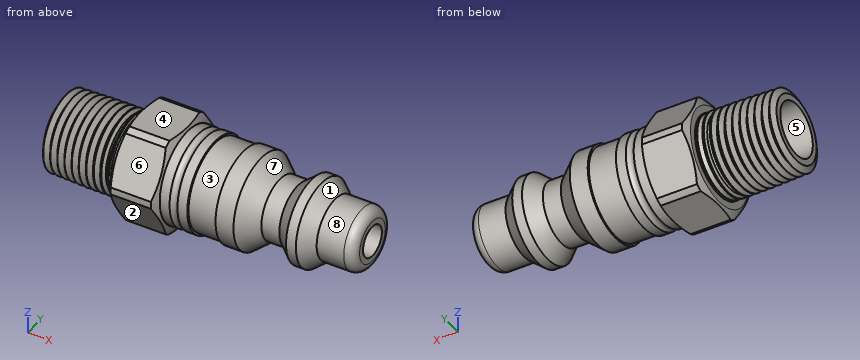
```python
from build123d import *

# Parameters (mm, degrees)
SKETCH6_W      = 11.300333551
SKETCH6_H      = 15.496408613
EXTRUDE1_DEPTH = 6.13324
FILLET1_R      = 1.27


with BuildPart() as part:
    # Sketch1 → Revolve1 (revolve)
    with BuildSketch(Plane.XY):
        Polygon((0, 0), (0, 4.202548436), (0.016953331, 4.234153018), (0.42773912, 4.999944315), (0.463586157, 5.001064591), (0.921387979, 4.262418014), (0.957235016, 4.26353829), (1.368020805, 5.029329586), (1.403867842, 5.030449862), (1.861669664, 4.291803285), (1.897516701, 4.292923561), (2.30830249, 5.058714857), (2.344149527, 5.059835133), (2.801951349, 4.321188556), (2.837798386, 4.322308832), (3.248584175, 5.088100128), (3.284431212, 5.089220404), (3.742233034, 4.350573827), (3.778080071, 4.351694103), (4.18886586, 5.1174854), (4.224712897, 5.118605675), (4.682514719, 4.379959098), (4.718361756, 4.381079374), (5.129147545, 5.146870671), (5.164994582, 5.147990947), (5.622796404, 4.409344369), (5.658643441, 4.410464645), (6.06942923, 5.176255942), (6.105276267, 5.177376218), (6.563078089, 4.43872964), (6.598925126, 4.439849916), (7.009710915, 5.205641213), (7.045557952, 5.206761489), (7.503359774, 4.468114911), (7.539206811, 4.469235187), (7.9499926, 5.235026484), (7.985839637, 5.23614676), (8.443641459, 4.497500182), (8.479488496, 4.498620458), (8.890274285, 5.264411755), (8.926121322, 5.265532031), (9.383923144, 4.526885454), (9.419770181, 4.528005729), (9.83055597, 5.293797026), (9.866403007, 5.294917302), (10.324204829, 4.556270725), (10.360051866, 4.557391001), (10.770837655, 5.323182297), (10.806684692, 5.324302573), (11.264486514, 4.585655996), (11.300333551, 4.586776272), (11.300333551, 0), align=None)
    revolve(axis=Axis((0, 0, 0), (-1, 0, 0)))

    # Sketch5 → Cut-Revolve2 (revolve, cut)
    with BuildSketch(Plane.XY, mode=Mode.PRIVATE) as cut_revolve2_sk:
        Polygon((9.96696, 0), (9.96696, 5.298059865), (11.300333551, 5.339729871), (11.300333551, 0), align=None)
    revolve(cut_revolve2_sk.sketch.rotate(Axis((0, 0, 0), (-1, 0, 0)), 180), axis=Axis((0, 0, 0), (-1, 0, 0)), mode=Mode.SUBTRACT)

    # Sketch6 → Cut-Revolve3 (revolve, cut)
    with BuildSketch(Plane.XY, mode=Mode.PRIVATE) as cut_revolve3_sk:
        with Locations((5.650166776, 12.891704307)):
            Rectangle(SKETCH6_W, SKETCH6_H)
    revolve(cut_revolve3_sk.sketch.rotate(Axis((0, 0, 0), (1, 0, 0)), 180), axis=Axis((0, 0, 0), (1, 0, 0)), mode=Mode.SUBTRACT)

    # Sketch7 → Revolve2 (revolve)
    with BuildSketch(Plane.XY, mode=Mode.PRIVATE) as revolve2_sk:
        Polygon((6.7056, 4.202548436), (9.96696, 5.1435), (9.96696, 4.202548436), align=None)
    revolve(revolve2_sk.sketch.rotate(Axis((0, 0, 0), (1, 0, 0)), 180), axis=Axis((0, 0, 0), (1, 0, 0)))

    # Sketch8 → Extrude1 (add)
    with BuildSketch(Plane(origin=(9.96696, 0, 0), x_dir=(0, 0, -1), z_dir=(1, 0, 0))):
        Polygon((0, 7.332348419), (-6.35, 3.666174209), (-6.35, -3.666174209), (0, -7.332348419), (6.35, -3.666174209), (6.35, 3.666174209), align=None)
    extrude(amount=EXTRUDE1_DEPTH)

    # Sketch9 → Cut-Revolve4 (revolve, cut)
    with BuildSketch(Plane.XY, mode=Mode.PRIVATE) as cut_revolve4_sk:
        Polygon((16.1002, 6.062348419), (15.626431419, 7.078348419), (10.440728581, 7.078348419), (9.96696, 6.062348419), (9.96696, 7.332348419), (16.1002, 7.332348419), align=None)
    revolve(cut_revolve4_sk.sketch.rotate(Axis((0, 0, 0), (1, 0, 0)), 180), axis=Axis((0, 0, 0), (1, 0, 0)), mode=Mode.SUBTRACT)

    # Sketch10 → Revolve3 (revolve)
    with BuildSketch(Plane.XY):
        with BuildLine():
            Line((16.1002, 0), (39.9, 0))
            Line((39.9, 0), (39.9, 3.96875))
            Line((39.9, 3.96875), (35.1375, 3.96875))
            Line((35.1375, 3.96875), (33.362408616, 5.458228526))
            Line((33.362408616, 5.458228526), (32.092408616, 5.458228526))
            Line((32.092408616, 5.458228526), (30.317317232, 3.96875))
            Line((30.317317232, 3.96875), (28.0001, 3.96875))
            Line((28.0001, 3.96875), (25.619597791, 5.966228526))
            Line((25.619597791, 5.966228526), (23.302380559, 5.966228526))
            Line((23.302380559, 5.966228526), (23.302380559, 5.712228526))
            Line((23.302380559, 5.712228526), (19.6562, 5.712228526))
            Line((19.6562, 5.712228526), (19.6562, 5.966228526))
            Line((19.6562, 5.966228526), (18.3862, 5.966228526))
            ThreePointArc((18.3862, 5.966228526), (17.8782, 5.712228526), (17.3702, 5.966228526))
            Line((17.3702, 5.966228526), (16.1002, 5.966228526))
            Line((16.1002, 5.966228526), (16.1002, 0))
        make_face()
    revolve(axis=Axis((0, 0, 0), (-1, 0, 0)))

    # Fillet1
    fillet1_edges = [part.edges().sort_by_distance(p)[0] for p in [
        (39.9, -3.96875, 0),
    ]]
    fillet(fillet1_edges, radius=FILLET1_R)

    # Sketch11 → Cut-Revolve5 (revolve, cut)
    with BuildSketch(Plane.XY, mode=Mode.PRIVATE) as cut_revolve5_sk:
        Polygon((9.96696, 3.4163), (16.1002, 1.984375), (39.9, 1.984375), (39.9, 0), (6.7056, 0), (0, 0), (0, 3.4163), align=None)
    revolve(cut_revolve5_sk.sketch.rotate(Axis((0, 0, 0), (-1, 0, 0)), 180), axis=Axis((0, 0, 0), (-1, 0, 0)), mode=Mode.SUBTRACT)


solid = part.part
```
Model file for the job. Use its own axes, mm. Face numbers are marked on the shaded views. A direction names the side the tool comes from. Coordinates: 2 decimals unless noted, no trailing zeros. Order: outer loops, then holes, each group sorted by start corner. A loop starts at its lowest first (then second) coordinate and runs counter-clockwise, first axis right, second up. Notation, with made-up numbers: (41.25, 6.5) -> (49.25, 6.5) arc R20 cw to (49.25, 35.5) -> close; hole circle Ø5 at (-10.75, 23). An arc over 180 degrees is marked (long way). Answer as a JSON object with one key per item and string values. Group by question number.
1) Pull direction X, two halves, no side cores. Call the marked faces 1, 2 and 3: +X half, -X half, draft (parallel to the pull), parting line (faces both ways), or undercut.
2) Which spindle directions (+Z, -Z, +X, -X, +Y, -Y) get a long thin tool onto all of the face, cutting with end or side? Do the marked faces 4, 5, 6, 7 and 8. Say none if no direction does.
3) Drill centre lines: L1, parallel to Y at x = 32.5, z = 3.75; L2, parallel to X at y = -3.25, z = 2.5; L3, parallel to Y at x = 10, z = 1.75. Where is each one in solid material? Low to high.
4) Cut at C-C, the plane x = 26.5. Write the cut outline in (y, z).
5) Flat gauge pins, fed straight in: pin 1 (4 mm diameter, centred on x = 6.5, y = 4.5, fed in from -Z); pin 2 (1 mm diameter, centred on x = 29.5, y = 1.5, fed in from -Z); pin 3 (1 mm diameter, centred on y = 3.5, z = 4, fed in from -X). Where does each tip first touch, or does it go through?
6) Cut at B-B, the plane x = 37.5. Write the cut outline in (y, z).
7) Cut at A-A, the plane x = 12. Write the cut outline in (y, z).
Check values:
{
 "1": {"face 1": "+X half", "face 2": "draft", "face 3": "undercut"},
 "2": {"face 4": "+Z, +X, -X, +Y, -Y", "face 5": "-X", "face 6": "+Z, +X, -X, -Y", "face 7": "none", "face 8": "+X"},
 "3": {"L1": "y = -3.97 to 3.97", "L2": "x = 0 to 27.84, 30.47 to 34.98", "L3": "y = -5.88 to -2.93, 2.93 to 5.88"},
 "4": {"outline": "circle Ø10.45 at (0, 0); hole circle Ø3.97 at (0, 0)"},
 "5": {"pin 1": "stops at z = -4.48", "pin 2": "stops at z = -3.84", "pin 3": "stops at x = 0.33"},
 "6": {"outline": "circle Ø7.94 at (0, 0); hole circle Ø3.97 at (0, 0)"},
 "7": {"outline": "(-7.06, -0.47) -> (-3.94, -5.88) arc R7.08 ccw to (-3.13, -6.35) -> (3.13, -6.35) arc R7.08 ccw to (3.94, -5.88) -> (7.06, -0.47) arc R7.08 ccw to (7.06, 0.47) -> (3.94, 5.88) arc R7.08 ccw to (3.13, 6.35) -> (-3.13, 6.35) arc R7.08 ccw to (-3.94, 5.88) -> (-7.06, 0.47) arc R7.08 ccw to start; hole circle Ø5.88 at (0, 0)"}
}
